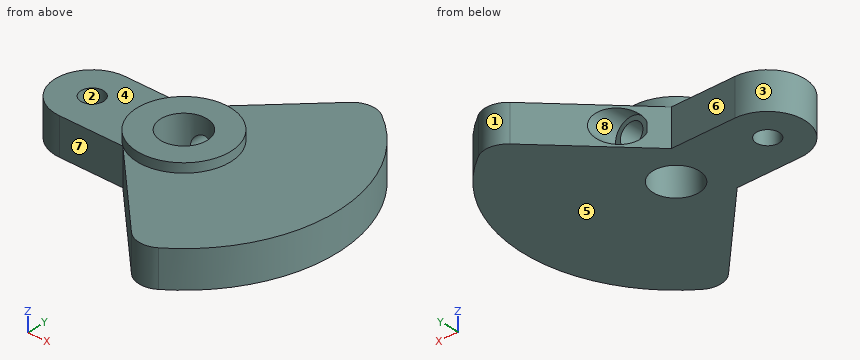
Autodesk Inventor part; units mm, degrees
ref_plane "Arbeitsebene1" through (0, 10, 0) normal (0, 1, 0) x (-1, 0, 0)
ref_plane "YZ Plane" through (0, 0, 0) normal (1, 0, 0) x (0, 1, 0)
ref_plane "XZ Plane" through (0, 0, 0) normal (0, 1, 0) x (-1, 0, 0)
sketch "Skizze1" plane through (0, 0, 0) normal (0, 0, 1) x (1, 0, 0)
  line L0 (0, -20.5159) -> (0, 20.5159)
  line L1 (-20.1, 0) -> (22.6, 0)
  circle A0 centre (0, 0) radius 2.5
  arc A1 (-3, 4) -> (-3, -4) centre (0, 0) ccw
  arc A2 (7.5831, -14.6542) -> (7.5831, 14.6542) centre (0, 0) ccw
  line L2 (-3.5355, 3.5355) -> (7.5831, 14.6542)
  line L3 (-3.5355, -3.5355) -> (7.5831, -14.6542)
  line L4 (-3, 4) -> (-10, 4)
  line L5 (-3, -4) -> (-10, -4)
  arc A3 (-10, 4) -> (-10, -4) centre (-10, 0) ccw
  dimension "d0" = 5
  dimension "d1" = 10
  dimension "d3" = 33
  dimension "d4" = 90
  dimension "d5" = 4
  dimension "d6" = 10
extrude "Extrusion1" add sketch "Skizze1" along normal blind 4 contours L3 L5 A1 L1 A0 L0 | L0 A0 L1 A2 L3 | L5 A3 L1 A1 L3 | L3 A1 L5 | L1 A1 L4 L2 L0 A0 | A0 L0 L2 A2 L1 | L1 A3 L4 L2 A1 | L2 L4 A1
fillet "Rundung1" radius 2.5 2 edges at (7.5831, 14.6542, 2) (7.5831, -14.6542, 2)
sketch "Skizze2" plane through (0, 0, 4) normal (0, 0, 1) x (1, 0, 0)
  arc A0 (-10, 4) -> (-10, -4) centre (-10, 0) ccw
  line L0 (0, -20.5159) -> (0, 20.5159)
  point P0 (0, 0)
hole "Bohrung1" at (-10, 0, 4) direction (0, 0, -1) diameter 2.459 end through all
sketch "Skizze3" plane through (0, 0, 4) normal (0, 0, 1) x (1, 0, 0)
  line L0 (0, -20.5159) -> (0, 20.5159)
  line L1 (-20.1, 0) -> (22.6, 0)
  line L2 (-10, -4) -> (-3.0711, -4)
  circle A0 centre (0, 0) radius 5.043
  circle A1 centre (0, 0) radius 2.5
  dimension "d17" = 5
extrude "Extrusion2" add sketch "Skizze3" along normal blind 1 contours A0 L1 A1 L0 | L0 A1 L1 A0 | L1 A1 L0 A0 | L1 A0 L0 A1
ref_plane "Arbeitsebene1" through (0, 10, 0) normal (0, 1, 0) x (-1, 0, 0)
sketch "Skizze7" plane through (0, 10, 0) normal (0, 1, 0) x (-1, 0, 0)
  line L0 (0, -0.8) -> (0, 4.8)
  line L1 (15, 0) -> (-2.5, 0)
  line L2 (10, 0) -> (10, 4)
  point P0 (0, 0)
  point P1 (0, 2)
  dimension "d30" = 2
hole "Bohrung3" at (0, 10, 2) direction (0, -1, 0) diameter 3.5 depth 4.6
sketch "Skizze8" plane through (0, 5.4, 2) normal (0, 1, 0) x (1, 0, 0)
  line L0 (0, 3) -> (0, -4)
  line L1 (22.6, 2) -> (-20.1, 2)
  point P0 (0, 2)
  point P1 (0, 0)
  dimension "d38" = 2
hole "Bohrung4" at (0, 5.4, 2) direction (0, -1, 0) diameter 2.459 end up to surface
properties part number "Kurbel 19"
For this review, take the finished solid that the model builds, in its own axes (mm). Face numbers are marked on the shaded views. A direction names the side the tool comes from. Round coordinates to 2 decimals unless told otherwise and drop trailing zeros. Write each loop counter-clockwise with the first axis right and the second up, starting at its lowest first coordinate (ties: lowest second). Pieces come first, ordered by that corner, then holes. Notation, with made-up numbers: (64.25, 88) - (92.25, 88) arc R27 cw to (92.25, 111) - close; hole circle Ø3 at (-35, -39.5). An arc over 180 degrees is marked (long way). Write each question's results on one line, items separated by ' | '.
Item 1: Take a section at C-C on x = 0. State the section outline as (y, z) points, then the cut area to 3 significant figures.
Calculated:
outline: (-7.07, 0) - (-2.5, 0) - (-2.5, 5) - (-5.04, 5) - (-5.04, 4) - (-7.07, 4) - close; (2.5, 0) - (7.07, 0) - (7.07, 0.25) - (5.4, 0.25) - (5.4, 0.77) - (2.5, 0.77) - close; (2.5, 3.23) - (5.4, 3.23) - (5.4, 3.75) - (7.07, 3.75) - (7.07, 4) - (5.04, 4) - (5.04, 5) - (2.5, 5) - close | area: 28.7 mm^2
Item 2: Take a section at D-D on y = 3. State the section outline as (x, z) points.
Calculated:
outline: (-12.65, 0) - (16.22, 0) - (16.22, 4) - (4.05, 4) - (4.05, 5) - (-4.05, 5) - (-4.05, 4) - (-12.65, 4) - close; hole circle Ø2.46 at (0, 2)
Item 3: For the marked faces 5, 6, 7 and 8, list the 3-axis set-ups (+Z, -Z, +X, -X, +Y, -Y) from which the entire face can be reached by the end or side of a thin tool; tool diameter is ignored.
Calculated:
face 5: -Z, +X, -X, +Y, -Y | face 6: +Z, -Z, -X, +Y | face 7: +Z, -Z, -X, -Y | face 8: +Y
Item 4: Take a section at B-B on z = 2. State the section outline as (x, y) points.
Calculated:
outline: (-10, -4) - (-3.07, -4) - (6.2, -13.28) arc R2.5 ccw to (9.4, -13.56) arc R16.5 ccw to (9.4, 13.56) arc R2.5 ccw to (6.2, 13.28) - (1.75, 8.82) - (1.75, 5.4) - (1.23, 5.4) - (1.23, 2.18) arc R2.5 cw (long way) to (-1.23, 2.18) - (-1.23, 5.4) - (-1.67, 5.4) - (-3.07, 4) - (-10, 4) arc R4 ccw to start; hole circle Ø2.46 at (-10, 0)
Item 5: For pin 1 (1.7 mm diameter, centred on x = 0, z = 2, fed in from +Y); pin 2 (2 mm diameter, centred on x = -7, z = 1.5, fed in from +Y); pin 3 (3 mm diameter, centred on x = -7, z = 1.5, fed in from -Y), all flat-tipped, find the tip position at first contact; note any pin that passes through.
Calculated:
pin 1: stops at y = -2.35 | pin 2: stops at y = 4 | pin 3: stops at y = -4
Item 6: To check wall thickness, follow line 1 along X through (y, z) = (0, 2.15); line 2 along Z through (x, y) = (0, 3.6); line 3 along Z through (x, y) = (11, -1). State the ranges of each line that lie inside material, in increasing order. Write a range as from..to.
Calculated:
line 1: x = -14..-11.23, -8.77..-2.5, 2.5..16.5 | line 2: z = 0..0.77, 3.23..5 | line 3: z = 0..4
Item 7: Take a section at A-A on y = 0. State the section outline as (x, z) points, then the cut area to 4 significant figures.
Calculated:
outline: (-14, 0) - (-11.23, 0) - (-11.23, 4) - (-14, 4) - close; (-8.77, 0) - (-2.5, 0) - (-2.5, 5) - (-5.04, 5) - (-5.04, 4) - (-8.77, 4) - close; (2.5, 0) - (16.5, 0) - (16.5, 4) - (5.04, 4) - (5.04, 5) - (2.5, 5) - close | area: 97.25 mm^2
Item 8: Draft analysis for pull direction Y (two halves, no side actions). For the marked faces 1, 2, 3 and 4, state which applies: pulls with the +Y half, pulls with the -Y half, needs draft (parallel to the pull), parting line crosses it, or undercut.
Calculated:
face 1: pulls with the +Y half | face 2: undercut | face 3: parting line crosses it | face 4: needs draft
